Can you work these out from the model? Positions are in its coordinate system, mm. A direction names the side the tool comes from. Give positions to 0.01 mm unless a question says otherwise; leave off trailing zeros. Order: outer loops, then holes, each group sorted by start corner. A loop starts at its lowest first (then second) coordinate and runs counter-clockwise, first axis right, second up. Notation, with made-up numbers: (51.5, -20) - (63.5, -20) arc R29 cw to (63.5, 10) - close; hole circle Ø11 at (74, 51.5). An arc over 180 degrees is marked (long way). Use one line per item in the form item = value. Start each with the question number.
1) Suppose I cut it at A-A, the plane x = -1. Write out the boundary of the cut face in (y, z), and give its area (3 significant figures).
2) For pin 1 (1.5 mm diameter, centred on y = 3, z = -2, fed in from -X); pin 2 (0.5 mm diameter, centred on y = 3.5, z = 6.5, fed in from -X); pin 3 (1.2 mm diameter, centred on y = 3.5, z = 6.09, fed in from +X); pin 4 (2 mm diameter, centred on x = 14, z = -4.5, fed in from +Y), each with a flat end and sliding along its axis, tell me the tip position at first contact or that it passes through.
3) Which directions (+Z, -Z, +X, -X, +Y, -Y) give clear straight access to the entire face, cutting with the end or side of a thin tool? Please do faces 5 (the cylindrical face through (-13.972, 2.228, -6.338)), 6 (the cylindrical face through (13.97, 2.88, 2.5)), 7 (the flat face through (14, 4.25, -4)).
4) Suppose I cut it at C-C, the plane y = 6. Write out the boundary of the cut face in (x, z).
5) Suppose I cut it at B-B, the plane z = -5. Write out the boundary of the cut face in (x, y).
6) We'd pull the mould along X, two halves only. Please class faces 1 (the cylindrical face through (-11.43, 0.6, -0.1)), 2 (the cylindrical face through (-11.43, 3.48, -8.4)), 3 (the flat face through (16, 4, -4)), 4 (the flat face through (0, 3, -9)): released by +X, released by -X, zero draft, split by the parting line, or undercut.
7) Suppose I cut it at D-D, the plane y = 3.5. State how many separate pieces and enclosed holes the cut face has, and give its area (3 significant figures).
8) Please list where these lines run through material, in increasing order: probe 1 along Y at (x, z) = (-13.8, -7); probe 2 along X at (y, z) = (3, -4); probe 3 along Y at (x, z) = (-13.5, 0.75).
```python
from build123d import *

# Parameters (mm, degrees)
BOSS_EXTRUDE1_DEPTH = 7
FILLET1_R           = 2
SKETCH2_R           = 1.434229719
SKETCH2_R_2         = 1.034229719
BOSS_EXTRUDE2_DEPTH = 4
SKETCH3_R           = 1.423607329
SKETCH3_R_2         = 1.023607329
SKETCH3_W           = 4.5
SKETCH3_H           = 1.5
BOSS_EXTRUDE3_DEPTH = 4


with BuildPart() as part:
    # Sketch1 → Boss-Extrude1 (new body)
    with BuildSketch(Plane(origin=(0, 0, 0), x_dir=(1, 0, 0), z_dir=(0, 1, 0))):
        with BuildLine():
            Line((-10, 9), (10, 9))
            ThreePointArc((10, 9), (11.414213562, 8.414213562), (12, 7))
            Line((12, 7), (12, -7))
            ThreePointArc((12, -7), (11.414213562, -8.414213562), (10, -9))
            Line((10, -9), (-10, -9))
            ThreePointArc((-10, -9), (-11.414213562, -8.414213562), (-12, -7))
            Line((-12, -7), (-12, 7))
            ThreePointArc((-12, 7), (-11.414213562, 8.414213562), (-10, 9))
        make_face()
    extrude(amount=BOSS_EXTRUDE1_DEPTH)

    # Fillet1
    fillet1_edges = [part.edges().sort_by_distance(p)[0] for p in [
        (0, 0, -9),
        (11.414213562, 0, -8.414213562),
        (12, 0, 0),
        (11.414213562, 0, 8.414213562),
        (11.414213562, 7, -8.414213562),
        (0, 7, -9),
        (-11.414213562, 7, -8.414213562),
        (-12, 7, 0),
        (-11.414213562, 7, 8.414213562),
        (0, 7, 9),
        (11.414213562, 7, 8.414213562),
        (0, 0, 9),
        (12, 7, 0),
        (-11.414213562, 0, 8.414213562),
        (-12, 0, 0),
        (-11.414213562, 0, -8.414213562),
    ]]
    fillet(fillet1_edges, radius=FILLET1_R)

    # Sketch2 → Boss-Extrude2 (add)
    with BuildSketch(Plane.ZY.offset(12)):
        with Locations((-7, 3.5)):
            Circle(SKETCH2_R)
        with Locations((-7, 3.5)):
            Circle(SKETCH2_R_2, mode=Mode.SUBTRACT)
        with Locations((0, 3.5)):
            Circle(SKETCH2_R)
        with Locations((0, 3.5)):
            Circle(SKETCH2_R_2, mode=Mode.SUBTRACT)
        with Locations((7, 3.5)):
            Circle(SKETCH2_R)
        with Locations((7, 3.5)):
            Circle(SKETCH2_R_2, mode=Mode.SUBTRACT)
    extrude(amount=BOSS_EXTRUDE2_DEPTH)

    # Sketch3 → Boss-Extrude3 (add)
    with BuildSketch(Plane(origin=(12, 0, 0), x_dir=(0, 0, -1), z_dir=(1, 0, 0))):
        with Locations((-6.085184826, 3.5)):
            Circle(SKETCH3_R)
        with Locations((-6.085184826, 3.5)):
            Circle(SKETCH3_R_2, mode=Mode.SUBTRACT)
        with Locations((-1.685184826, 3.5)):
            Circle(SKETCH3_R)
        with Locations((-1.685184826, 3.5)):
            Circle(SKETCH3_R_2, mode=Mode.SUBTRACT)
        with Locations((4.044962508, 3.5)):
            Rectangle(SKETCH3_W, SKETCH3_H)
    extrude(amount=BOSS_EXTRUDE3_DEPTH)


solid = part.part
```
Result sheet:
q1.outline = (0, -7) arc R2 ccw to (2, -9) - (5, -9) arc R2 ccw to (7, -7) - (7, 7) arc R2 ccw to (5, 9) - (2, 9) arc R2 ccw to (0, 7) - close
q1.area = 123 mm²
q2.pin_1 = -16
q2.pin_2 = -12
q2.pin_3 = 12
q2.pin_4 = 4.25
q3.face_5 = -X
q3.face_6 = +X
q3.face_7 = -Z, +X, +Y
q4.outline = (-11.73, -7) arc R1.73 ccw to (-10, -8.73) - (10, -8.73) arc R1.73 ccw to (11.73, -7) - (11.73, 7) arc R1.73 ccw to (10, 8.73) - (-10, 8.73) arc R1.73 ccw to (-11.73, 7) - close
q5.outline = (-12, 2) arc R2 ccw to (-10, 0) - (10, 0) arc R2 ccw to (12, 2) - (12, 2.75) - (16, 2.75) - (16, 4.25) - (12, 4.25) - (12, 5) arc R2 ccw to (10, 7) - (-10, 7) arc R2 ccw to (-12, 5) - close
q6.face_1 = released by -X
q6.face_2 = undercut
q6.face_3 = released by +X
q6.face_4 = zero draft
q7.separate_pieces = 4
q7.enclosed_holes = 0
q7.area = 463 mm²
q8.probe_1 = 2.07 to 2.47, 4.53 to 4.93
q8.probe_2 = -12 to 16
q8.probe_3 = 2.28 to 2.79, 4.21 to 4.72
